Autodesk Inventor part; units mm, degrees
ref_plane "YZ Plane" through (0, 0, 0) normal (1, 0, 0) x (0, 1, 0)
ref_plane "XZ Plane" through (0, 0, 0) normal (0, 1, 0) x (-1, 0, 0)
ref_plane "XY Plane" through (0, 0, 0) normal (0, 0, 1) x (1, 0, 0)
sketch "Esquisse1" plane through (0, 0, 0) normal (1, 0, 0) x (0, 1, 0)
  line L0 (9.85, 20.25) -> (-9.85, 20.25)
  line L1 (-9.85, 20.25) -> (-9.85, -20.25)
  line L2 (-9.85, -20.25) -> (9.85, -20.25)
  line L3 (9.85, -20.25) -> (9.85, 20.25)
  line L4 (9.85, 20.25) -> (-9.85, -20.25)
  line L5 (-9.85, 20.25) -> (9.85, -20.25)
  point P0 (0, 0)
  point P1 (0, 0)
  point P2 (0, 0)
  dimension "d0" = 19.7
  dimension "d1" = 40.5
extrude "Extrusion1" add sketch "Esquisse1" along normal blind 38
sketch "Esquisse2" plane through (0, -9.85, -20.25) normal (0, 0, -1) x (-1, 0, 0)
  line L0 (0, 0) -> (-38, 0)
  line L1 (0, 19.7) -> (-38, 19.7)
  line L2 (-32.8, 0) -> (-30.4, 0)
  line L3 (-30.4, 0) -> (-30.4, 19.7)
  line L4 (-30.4, 19.7) -> (-32.8, 19.7)
  line L5 (-32.8, 19.7) -> (-32.8, 0)
  line L6 (-38, 0) -> (-38, 19.7)
  point P0 (0, 9.85)
  dimension "d4" = 5.2
  dimension "d5" = 2.4
extrude "Extrusion2" add sketch "Esquisse2" along normal blind 7.2 contours L0 L5 L1 L3
sketch "Esquisse3" plane through (0, -9.85, 20.25) normal (0, 0, 1) x (1, 0, 0)
  line L0 (32.8, 19.7) -> (38, 19.7)
  line L1 (32.8, 19.7) -> (30.4, 19.7)
  line L2 (30.4, 19.7) -> (30.4, 0)
  line L3 (30.4, 0) -> (32.8, 0)
  line L4 (32.8, 0) -> (32.8, 19.7)
  point P0 (0, 9.85)
extrude "Extrusion3" add sketch "Esquisse3" along normal blind 7.2
sketch "Esquisse4" plane through (32.8, -9.85, 20.25) normal (1, 0, 0) x (0, 0, -1)
  line L0 (40.5, 19.7) -> (0, 19.7)
  line L1 (20.25, 19.7) -> (20.25, 0)
  line L2 (0, 0) -> (40.5, 0)
  circle A0 centre (-3.9, 14.85) radius 2.25
  line L3 (-7.2, 19.7) -> (-7.2, 0)
  line L4 (-7.2, 9.85) -> (47.7, 9.85)
  line L5 (47.7, 0) -> (47.7, 19.7)
  circle A1 centre (-3.9, 4.85) radius 2.25
  circle A2 centre (44.4, 14.85) radius 2.25
  circle A3 centre (44.4, 4.85) radius 2.25
  point P0 (20.25, 9.85)
  dimension "d10" = 4.5
  dimension "d11" = 10
  dimension "d19" = 24.15
extrude "Extrusion4" cut sketch "Esquisse4" against normal blind 7.2
sketch "Esquisse5" plane through (38, 0, 0) normal (1, 0, 0) x (0, 0, -1)
  circle A0 centre (-10, 0) radius 6
  point P0 (0, 0)
  dimension "d14" = 12
  dimension "d15" = 10
extrude "Extrusion5" add sketch "Esquisse5" along normal blind 7.2
fillet "Congé1" radius 5 2 edges at (0, 0, 20.25) (0, 0, -20.25)
properties part number "servomoteur_roues"
Can you work these out from the model? Positions are in its coordinate system, mm. A direction names the side the tool comes from. Round coordinates to 2 decimals unless told otherwise and drop trailing zeros. Loops run counter-clockwise (first coordinate to the right, second up) from the corner with the lowest first, then second, coordinate; pieces in that order, holes last.
Item 1: Suppose I cut it at A-A, the plane z = 10. Write out the boundary of the cut face in (x, y).
Item 2: Will these pins go through, and if not, where does the flat tip stop? pin 1 Ø5 at (y, z) = (5, 24.15) entering from -X; pin 2 Ø8 at (y, z) = (-0.5, -22.5) entering from -X; pin 3 Ø6 at (y, z) = (-6.5, 0) entering from +X; pin 4 Ø3.5 at (y, z) = (-5, 24.15) entering from +X.
Item 3: Suppose I cut it at B-B, the plane y = 5. Write out the boundary of the cut face in (x, z).
Item 4: Please list where these lines run through material, in increasing order: L1, parallel to Y at x = 31, z = 24 (3 decimals); L2, parallel to Z at x = 12, y = 1; L3, parallel to X at y = -3, z = 21.
Item 5: If we mould it in two halves opening along Y, with no side actions, what happens to faces 5 (the cylindrical face through (1.5, 0.14, -18.82)), 6 (the cylindrical face through (31.617, -4.324, -26.296)), 7 (the flat face through (19, -9.85, 0))? For each: +Y half, -Y half, draft (parallel to the pull), parting line (faces both ways), or undercut.
Item 6: Suppose I cut it at C-C, the plane z = 24.15. Write out the boundary of the cut face in (x, y).
Item 7: Which directions (+Z, -Z, +X, -X, +Y, -Y) give clear straight access to the entire face, cutting with the end or side of a thin tool? Please do faces 1 (the flat face through (18, 0, -20.25)), 2 (the flat face through (18, 0, 20.25)), 3 (the flat face through (35, 0, 20.25)), 4 (the flat face through (35, 0, -20.25)).
Item 8: Suppose I cut it at D-D, the plane y = 0. Write out the boundary of the cut face in (x, z).
Reported:
1. outline: (0, -9.85) - (38, -9.85) - (38, -6) - (45.2, -6) - (45.2, 6) - (38, 6) - (38, 9.85) - (0, 9.85) - close
2. pin 1: stops at x = 30.4
2. pin 2: stops at x = 1.2
2. pin 3: stops at x = 38
2. pin 4: passes through
3. outline: (0, -15.25) arc R5 ccw to (5, -20.25) - (30.4, -20.25) - (30.4, -21.9) - (32.8, -21.9) - (32.8, -20.25) - (38, -20.25) - (38, 6.68) - (45.2, 6.68) - (45.2, 13.32) - (38, 13.32) - (38, 20.25) - (32.8, 20.25) - (32.8, 21.9) - (30.4, 21.9) - (30.4, 20.25) - (5, 20.25) arc R5 ccw to (0, 15.25) - close; (30.4, -27.45) - (32.8, -27.45) - (32.8, -26.4) - (30.4, -26.4) - close; (30.4, 26.4) - (32.8, 26.4) - (32.8, 27.45) - (30.4, 27.45) - close
4. L1: y = -9.85 to -7.245, -2.755 to 2.755, 7.245 to 9.85
4. L2: z = -20.25 to 20.25
4. L3: x = 30.4 to 32.8
5. face 5: draft
5. face 6: undercut
5. face 7: -Y half
6. outline: (30.4, -9.85) - (32.8, -9.85) - (32.8, -7.25) - (30.4, -7.25) - close; (30.4, -2.75) - (32.8, -2.75) - (32.8, 2.75) - (30.4, 2.75) - close; (30.4, 7.25) - (32.8, 7.25) - (32.8, 9.85) - (30.4, 9.85) - close
7. face 1: -Z, -X, +Y, -Y
7. face 2: +Z, -X, +Y, -Y
7. face 3: +Z, +X, +Y, -Y
7. face 4: -Z, +X, +Y, -Y
8. outline: (0, -15.25) arc R5 ccw to (5, -20.25) - (30.4, -20.25) - (30.4, -27.45) - (32.8, -27.45) - (32.8, -20.25) - (38, -20.25) - (38, 4) - (45.2, 4) - (45.2, 16) - (38, 16) - (38, 20.25) - (32.8, 20.25) - (32.8, 27.45) - (30.4, 27.45) - (30.4, 20.25) - (5, 20.25) arc R5 ccw to (0, 15.25) - close
